The model under review builds one solid part; all positions refer to its coordinate system, in mm. A direction names the side the tool comes from. Give positions to 0.01 mm unless a question says otherwise; leave off trailing zeros. Order: outer loops, then holes, each group sorted by start corner. A loop starts at its lowest first (then second) coordinate and runs counter-clockwise, first axis right, second up. Notation, with made-up numbers: (-13.75, -23.75) -> (-5.75, -23.75) arc R27 cw to (-5.75, 5.25) -> close; hole circle Ø5 at (85.5, 71). An arc over 180 degrees is marked (long way). Use one line per item in the form item = value.
```python
from build123d import *

# Parameters (mm, degrees)
F1_DEPTH = 0.5
F2_R     = 22
F3_DEPTH = 0.85
F4_R     = 22
F5_DEPTH = 0.85


with BuildPart() as f1:
    # F0 (on Top) → F1 (new body)
    with BuildSketch(Plane.XY):
        with BuildLine():
            Line((24, -7), (24, 7))
            ThreePointArc((24, 7), (0, 25), (-24, 7))
            Line((-24, 7), (-24, -7))
            ThreePointArc((-24, -7), (0, -25), (24, -7))
        make_face()
    extrude(amount=F1_DEPTH)

    # F2 (on face) → F3 (join)
    with BuildSketch(Plane.XY.offset(0.5)):
        with BuildLine():
            ThreePointArc((-24, -7), (0, -25), (24, -7))
            Line((24, -7), (24, 7))
            ThreePointArc((24, 7), (0, 25), (-24, 7))
            Line((-24, 7), (-24, -7))
        make_face()
        Circle(F2_R, mode=Mode.SUBTRACT)
    extrude(amount=F3_DEPTH)

    # F4 (on face) → F5 (join)
    with BuildSketch(Plane(origin=(0, 0, 0), x_dir=(1, 0, 0), z_dir=(0, 0, -1))):
        with BuildLine():
            ThreePointArc((24, 7), (0, 25), (-24, 7))
            Line((-24, 7), (-24, -7))
            ThreePointArc((-24, -7), (0, -25), (24, -7))
            Line((24, -7), (24, 7))
        make_face()
        Circle(F4_R, mode=Mode.SUBTRACT)
    extrude(amount=F5_DEPTH)


solid = f1.part
```
1. The part is to be moulded in two halves that separate along Y. For faces 1 (the face through (24, 0, 0)), 2 (the face through (-4.769, -21.477, 0.919)), 3 (the face through (0, 25, 0)), say which applies: +Y half, -Y half, draft (parallel to the pull), parting line (faces both ways), or undercut.
Values:
face_1 = draft
face_2 = undercut
face_3 = +Y half
2. For L1, parallel to Y at x = 0, z = -0.6; L2, parallel to X at y = 0, z = -0.35; L3, parallel to Z at x = -1, y = 15, list the stretches that pass through material, from the lowest coordinate up.
Values:
L1 = -25 to -22, 22 to 25
L2 = -24 to -22, 22 to 24
L3 = 0 to 0.5
3. For pin 1 Ø22 at (x, y) = (-3.5, 10.5) entering from +Z; pin 2 Ø1 at (x, z) = (5.5, 0) entering from +Y; pin 3 Ø1 at (x, y) = (0, -15.5) entering from +Z; pin 4 Ø1 at (x, y) = (14, 12.5) entering from -Z, all flat-tipped, find the tip position at first contact; note any pin that passes through.
Values:
pin_1 = 1.35
pin_2 = 24.49
pin_3 = 0.5
pin_4 = 0
4. Add section B-B on x = 0. Give the boundary of the cut face in (y, z), then the cut area to 3 significant figures.
Values:
outline = (-25, -0.85) -> (-22, -0.85) -> (-22, 0) -> (22, 0) -> (22, -0.85) -> (25, -0.85) -> (25, 1.35) -> (22, 1.35) -> (22, 0.5) -> (-22, 0.5) -> (-22, 1.35) -> (-25, 1.35) -> close
area = 35.2 mm^2
5. Add section A-A on y = 0. Give the boundary of the cut face in (x, z).
Values:
outline = (-24, -0.85) -> (-22, -0.85) -> (-22, 0) -> (22, 0) -> (22, -0.85) -> (24, -0.85) -> (24, 1.35) -> (22, 1.35) -> (22, 0.5) -> (-22, 0.5) -> (-22, 1.35) -> (-24, 1.35) -> close
6. Tool access review of faces 4 (the face through (-9, -20.3, 1.35)), 5 (the face through (-4.769, 21.477, -0.419)), 6 (the face through (0, 0, 0.5)): name each direction out of +Z, -Z, +X, -X, +Y, -Y from which nothing blocks a thin tool from reaching the whole face with its end or side.
Values:
face_4 = +Z, +X, -X, +Y, -Y
face_5 = -Z
face_6 = +Z
